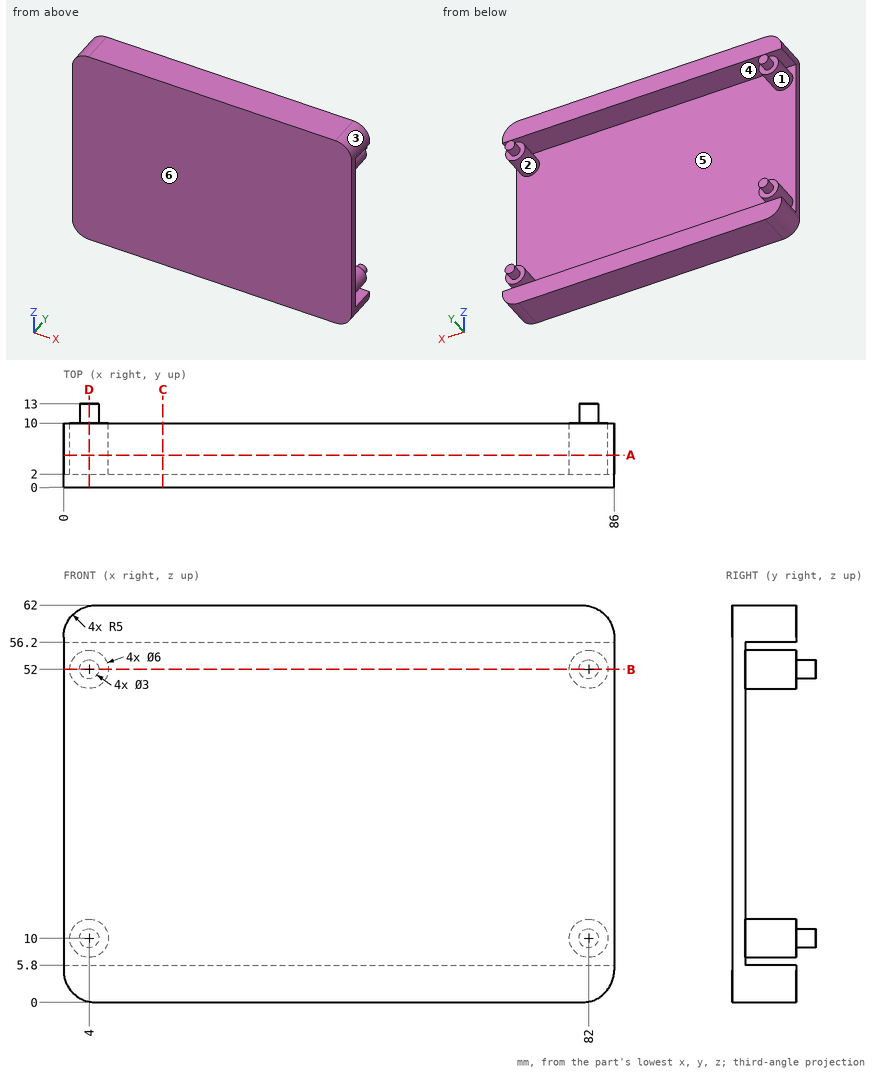
Input: dimensioned drawing with shaded views. Units: mm. Origin: part minimum x, y, z. A direction names the side the tool comes from. Give positions to 0.01 mm unless a question says otherwise; leave off trailing zeros. Write each loop counter-clockwise with the first axis right and the second up, starting at its lowest first coordinate (ties: lowest second). Pieces come first, ordered by that corner, then holes. Notation, with made-up numbers: M 29.25,6 L 79.25,6 A33 ccw 79.25,41 Z; hole C 77.25,76.25 d2. An arc over 180 degrees is marked long. Return JSON: item names as keys, results as strings. Group by question number.
1) Pull-direction query (X, two-part tool) for the marked faces 1, 2, 3 and 4; classes: pulls with the +X half, pulls with the -X half, needs draft (parallel to the pull), parting line crosses it, or undercut.
2) Pin query (flat end, axial travel): P1, Ø1, axis at x = 31.5, z = 12, coming from the +Y side; P2, Ø1.7, axis at x = 43, z = 57.5, coming from the +Y side. Return the tip coordinate at first contact, or that it passes through.
3) Set-up query: the marked faces 5 and 6. Return all of +Z, -Z, +X, -X, +Y, -Y with unobstructed straight access to the full face (end or side cutting, diameter ignored); none if empty.
4) Cut plane A-A, the plane y = 5. Output: boundary loops of the cut face in (x, z).
5) Cut plane B-B, the plane z = 52. Output: boundary loops of the cut face in (x, y).
6) Material intervals for line 1 along Z through (x, y) = (9, 2.5); line 2 along Y through (x, z) = (52, 56); line 3 along Y through (x, z) = (22, 3), sorted ascending. Write a range as [from, to].
7) Cut plane D-D, the plane x = 4. Output: boundary loops of the cut face in (y, z).
8) Cut plane C-C, the plane x = 15.5. Output: boundary loops of the cut face in (y, z).
Recorded:
{
 "1": {"face 1": "undercut", "face 2": "undercut", "face 3": "pulls with the +X half", "face 4": "needs draft"},
 "2": {"P1": "stops at y = 2", "P2": "stops at y = 10"},
 "3": {"face 5": "+Y", "face 6": "+Z, -Z, +X, -X, -Y"},
 "4": {"outline": "M 0,5 A5 ccw 5,0 L 81,0 A5 ccw 86,5 L 86,5.8 L 0,5.8 Z; M 0,56.2 L 86,56.2 L 86,57 A5 ccw 81,62 L 5,62 A5 ccw 0,57 Z; C 4,10 d6; C 4,52 d6; C 82,10 d6; C 82,52 d6"},
 "5": {"outline": "M 0,0 L 86,0 L 86,2 L 85,2 L 85,10 L 83.5,10 L 83.5,13 L 80.5,13 L 80.5,10 L 79,10 L 79,2 L 7,2 L 7,10 L 5.5,10 L 5.5,13 L 2.5,13 L 2.5,10 L 1,10 L 1,2 L 0,2 Z"},
 "6": {"line 1": "z = [0, 5.8], [56.2, 62]", "line 2": "y = [0, 2]", "line 3": "y = [0, 10]"},
 "7": {"outline": "M 0,0.1 L 10,0.1 L 10,5.8 L 2,5.8 L 2,7 L 10,7 L 10,8.5 L 13,8.5 L 13,11.5 L 10,11.5 L 10,13 L 2,13 L 2,49 L 10,49 L 10,50.5 L 13,50.5 L 13,53.5 L 10,53.5 L 10,55 L 2,55 L 2,56.2 L 10,56.2 L 10,61.9 L 0,61.9 Z"},
 "8": {"outline": "M 0,0 L 10,0 L 10,5.8 L 2,5.8 L 2,56.2 L 10,56.2 L 10,62 L 0,62 Z"}
}
